Geometry check sheet. Reference: drawing and pictorial views, mm from the part's lowest x, y, z. A direction names the side the tool comes from. Give positions to 0.01 mm unless a question says otherwise; leave off trailing zeros. Write each loop counter-clockwise with the first axis right and the second up, starting at its lowest first coordinate (ties: lowest second). Pieces come first, ordered by that corner, then holes. Notation, with made-up numbers: M -32.75,-26 L 20.25,-26 A16 cw 20.25,-10 Z; hole C -11.75,10 d4. An arc over 180 degrees is marked long. One line per item, written item: value. Start each with the question number.
1. Scan lines: line 1 (Z direction, x = 45, y = 35); line 2 (Z direction, x = 45, y = 42.5); line 3 (Y direction, x = 25, z = 6). Record each from-to range of solid material in increasing order.
2. Gauge pin test, flat ends, axial feed: pin 1 (2 mm diameter, centred on y = 41, z = 34.5, fed in from +X); pin 2 (8 mm diameter, centred on x = 45, z = 45, fed in from +Y); pin 3 (8 mm diameter, centred on y = 63, z = 45, fed in from +X); pin 4 (12 mm diameter, centred on x = 68, z = 68.5, fed in from +Y). Record the tip position at first contact, or that the pin passes through.
3. Tool access check on the marked faces 1, 2 and 3. Record the directions out of +Z, -Z, +X, -X, +Y, -Y that give a thin tool (end or side, any length) a straight path to the whole face; none if there is none.
4. Cross-section at A-A on z = 45. Record the cut outline in (x, y), then the cut area to 3 significant figures.
5. Cross-section at D-D on x = 27.5. Record the cut outline in (y, z), then the cut area to 3 significant figures.
6. Cross-section at B-B on y = 20. Record the cut outline in (x, z), then the cut area to 3 significant figures.
7. Cross-section at C-C on z = 114. Record the cut outline in (x, y), then the cut area to 3 significant figures.
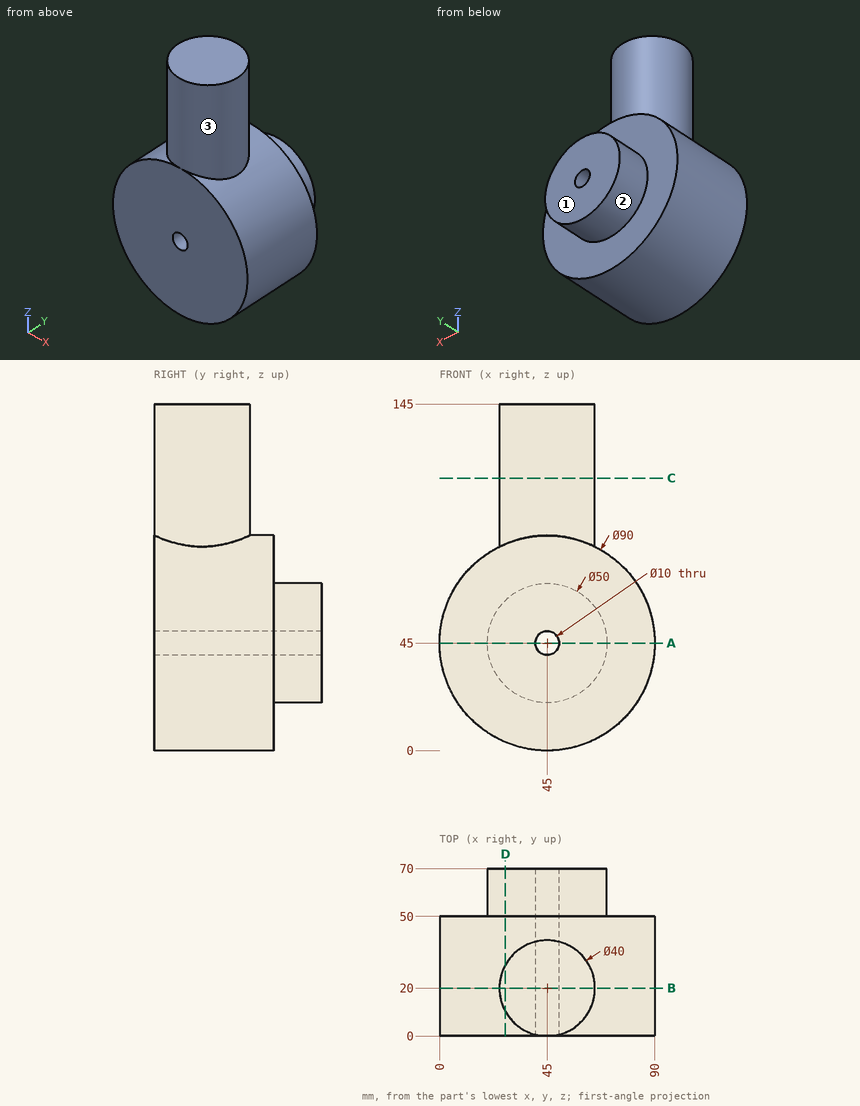
Report:
1. line 1: z = 0 to 40, 50 to 145
1. line 2: z = 0 to 40, 50 to 90
1. line 3: y = 0 to 50
2. pin 1: stops at x = 88.99
2. pin 2: passes through
2. pin 3: stops at x = 70
2. pin 4: stops at y = 50
3. face 1: +Z, -Z, +X, -X, +Y
3. face 2: +Y
3. face 3: +Z
4. outline: M 0,0 L 40,0 L 40,70 L 20,70 L 20,50 L 0,50 Z; M 50,0 L 90,0 L 90,50 L 70,50 L 70,70 L 50,70 Z
4. area: 4,800 mm^2
5. outline: M 0,3.54 L 50,3.54 L 50,27.15 L 70,27.15 L 70,62.85 L 50,62.85 L 50,86.46 L 29.68,86.46 L 29.68,145 L 10.32,145 L 10.32,86.46 L 0,86.46 Z
5. area: 5,990 mm^2
6. outline: M 25,85.31 A45 ccw long 65,85.31 L 65,145 L 25,145 Z; hole C 45,45 d10
6. area: 8,540 mm^2
7. outline: C 45,20 d40
7. area: 1,260 mm^2
